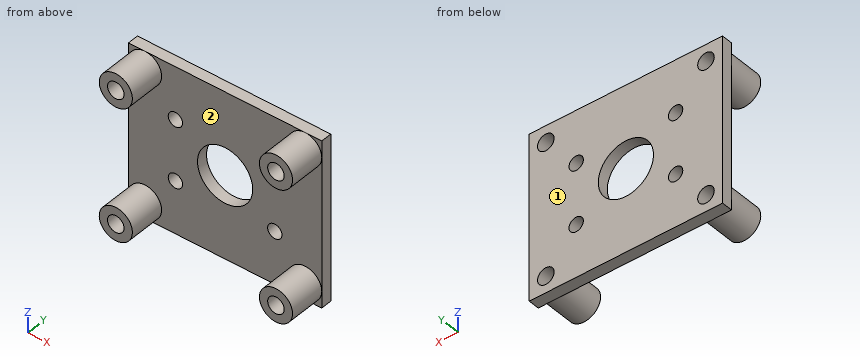
```python
from build123d import *

# Parameters (mm, degrees)
SKETCH1_W           = 35
SKETCH1_H           = 30
BOSS_EXTRUDE1_DEPTH = 2
CUT_EXTRUDE1_REACH  = 25.135
SKETCH2_R           = 1.3
CUT_EXTRUDE2_REACH  = 25.135
SKETCH3_R           = 1.5
SKETCH4_R           = 3
BOSS_EXTRUDE2_DEPTH = 6.5
CUT_EXTRUDE3_REACH  = 25.948
SKETCH5_R           = 1.5
SKETCH7_R           = 5
CUT_EXTRUDE4_DEPTH  = 3


with BuildPart() as part:
    # Sketch1 → Boss-Extrude1 (new body)
    with BuildSketch(Plane(origin=(0, 0, 0), x_dir=(1, 0, 0), z_dir=(0, 1, 0))):
        Rectangle(SKETCH1_W, SKETCH1_H)
    extrude(amount=BOSS_EXTRUDE1_DEPTH)

    # Sketch2 → Cut-Extrude1 (cut, up to next)
    with BuildSketch(Plane(origin=(0, 2, 0), x_dir=(1, 0, 0), z_dir=(0, 1, 0)), mode=Mode.PRIVATE) as cut_extrude1_sk1:
        with Locations(Location((9, 5.5, 0), (0, 0, 270))):
            Circle(SKETCH2_R)
    cut_extrude1_tool1 = extrude(cut_extrude1_sk1.sketch, amount=-CUT_EXTRUDE1_REACH, mode=Mode.PRIVATE) & part.part
    # Sketch2 → Cut-Extrude1 (cut, up to next)
    with BuildSketch(Plane(origin=(0, 2, 0), x_dir=(1, 0, 0), z_dir=(0, 1, 0)), mode=Mode.PRIVATE) as cut_extrude1_sk2:
        with Locations(Location((-9, 5.5, 0), (0, 0, 270))):
            Circle(SKETCH2_R)
    cut_extrude1_tool2 = extrude(cut_extrude1_sk2.sketch, amount=-CUT_EXTRUDE1_REACH, mode=Mode.PRIVATE) & part.part
    # Sketch2 → Cut-Extrude1 (cut, up to next)
    with BuildSketch(Plane(origin=(0, 2, 0), x_dir=(1, 0, 0), z_dir=(0, 1, 0)), mode=Mode.PRIVATE) as cut_extrude1_sk3:
        with Locations(Location((9, -5.5, 0), (0, 0, 270))):
            Circle(SKETCH2_R)
    cut_extrude1_tool3 = extrude(cut_extrude1_sk3.sketch, amount=-CUT_EXTRUDE1_REACH, mode=Mode.PRIVATE) & part.part
    # Sketch2 → Cut-Extrude1 (cut, up to next)
    with BuildSketch(Plane(origin=(0, 2, 0), x_dir=(1, 0, 0), z_dir=(0, 1, 0)), mode=Mode.PRIVATE) as cut_extrude1_sk4:
        with Locations(Location((-9, -5.5, 0), (0, 0, 270))):
            Circle(SKETCH2_R)
    cut_extrude1_tool4 = extrude(cut_extrude1_sk4.sketch, amount=-CUT_EXTRUDE1_REACH, mode=Mode.PRIVATE) & part.part
    add(cut_extrude1_tool1.solids().sort_by_distance((9, 2, -5.5))[0], mode=Mode.SUBTRACT)
    add(cut_extrude1_tool2.solids().sort_by_distance((-9, 2, -5.5))[0], mode=Mode.SUBTRACT)
    add(cut_extrude1_tool3.solids().sort_by_distance((9, 2, 5.5))[0], mode=Mode.SUBTRACT)
    add(cut_extrude1_tool4.solids().sort_by_distance((-9, 2, 5.5))[0], mode=Mode.SUBTRACT)

    # Sketch3 → Cut-Extrude2 (cut, up to next)
    with BuildSketch(Plane.XZ, mode=Mode.PRIVATE) as cut_extrude2_sk1:
        with Locations(Location((-14.5, 12, 0), (0, 0, 270))):
            Circle(SKETCH3_R)
    cut_extrude2_tool1 = extrude(cut_extrude2_sk1.sketch, amount=-CUT_EXTRUDE2_REACH, mode=Mode.PRIVATE) & part.part
    # Sketch3 → Cut-Extrude2 (cut, up to next)
    with BuildSketch(Plane.XZ, mode=Mode.PRIVATE) as cut_extrude2_sk2:
        with Locations(Location((14.5, 12, 0), (0, 0, 270))):
            Circle(SKETCH3_R)
    cut_extrude2_tool2 = extrude(cut_extrude2_sk2.sketch, amount=-CUT_EXTRUDE2_REACH, mode=Mode.PRIVATE) & part.part
    # Sketch3 → Cut-Extrude2 (cut, up to next)
    with BuildSketch(Plane.XZ, mode=Mode.PRIVATE) as cut_extrude2_sk3:
        with Locations(Location((14.5, -12, 0), (0, 0, 90))):
            Circle(SKETCH3_R)
    cut_extrude2_tool3 = extrude(cut_extrude2_sk3.sketch, amount=-CUT_EXTRUDE2_REACH, mode=Mode.PRIVATE) & part.part
    # Sketch3 → Cut-Extrude2 (cut, up to next)
    with BuildSketch(Plane.XZ, mode=Mode.PRIVATE) as cut_extrude2_sk4:
        with Locations(Location((-14.5, -12, 0), (0, 0, 90))):
            Circle(SKETCH3_R)
    cut_extrude2_tool4 = extrude(cut_extrude2_sk4.sketch, amount=-CUT_EXTRUDE2_REACH, mode=Mode.PRIVATE) & part.part
    add(cut_extrude2_tool1.solids().sort_by_distance((-14.5, 0, 12))[0], mode=Mode.SUBTRACT)
    add(cut_extrude2_tool2.solids().sort_by_distance((14.5, 0, 12))[0], mode=Mode.SUBTRACT)
    add(cut_extrude2_tool3.solids().sort_by_distance((14.5, 0, -12))[0], mode=Mode.SUBTRACT)
    add(cut_extrude2_tool4.solids().sort_by_distance((-14.5, 0, -12))[0], mode=Mode.SUBTRACT)

    # Sketch4 → Boss-Extrude2 (add)
    with BuildSketch(Plane.XZ):
        with Locations(Location((-14.5, 12, 0), (0, 0, 90))):
            Circle(SKETCH4_R)
        with Locations(Location((14.5, 12, 0), (0, 0, 90))):
            Circle(SKETCH4_R)
        with Locations(Location((-14.5, -12, 0), (0, 0, 270))):
            Circle(SKETCH4_R)
        with Locations(Location((14.5, -12, 0), (0, 0, 270))):
            Circle(SKETCH4_R)
    extrude(amount=BOSS_EXTRUDE2_DEPTH)

    # Sketch5 → Cut-Extrude3 (cut, up to next)
    with BuildSketch(Plane(origin=(0, 0, 0), x_dir=(1, 0, 0), z_dir=(0, 1, 0)), mode=Mode.PRIVATE) as cut_extrude3_sk1:
        with Locations(Location((-14.5, 12, 0), (0, 0, 90))):
            Circle(SKETCH5_R)
    cut_extrude3_tool1 = extrude(cut_extrude3_sk1.sketch, amount=-CUT_EXTRUDE3_REACH, mode=Mode.PRIVATE) & part.part
    # Sketch5 → Cut-Extrude3 (cut, up to next)
    with BuildSketch(Plane(origin=(0, 0, 0), x_dir=(1, 0, 0), z_dir=(0, 1, 0)), mode=Mode.PRIVATE) as cut_extrude3_sk2:
        with Locations(Location((14.5, 12, 0), (0, 0, 90))):
            Circle(SKETCH5_R)
    cut_extrude3_tool2 = extrude(cut_extrude3_sk2.sketch, amount=-CUT_EXTRUDE3_REACH, mode=Mode.PRIVATE) & part.part
    # Sketch5 → Cut-Extrude3 (cut, up to next)
    with BuildSketch(Plane(origin=(0, 0, 0), x_dir=(1, 0, 0), z_dir=(0, 1, 0)), mode=Mode.PRIVATE) as cut_extrude3_sk3:
        with Locations(Location((14.5, -12, 0), (0, 0, 90))):
            Circle(SKETCH5_R)
    cut_extrude3_tool3 = extrude(cut_extrude3_sk3.sketch, amount=-CUT_EXTRUDE3_REACH, mode=Mode.PRIVATE) & part.part
    # Sketch5 → Cut-Extrude3 (cut, up to next)
    with BuildSketch(Plane(origin=(0, 0, 0), x_dir=(1, 0, 0), z_dir=(0, 1, 0)), mode=Mode.PRIVATE) as cut_extrude3_sk4:
        with Locations(Location((-14.5, -12, 0), (0, 0, 90))):
            Circle(SKETCH5_R)
    cut_extrude3_tool4 = extrude(cut_extrude3_sk4.sketch, amount=-CUT_EXTRUDE3_REACH, mode=Mode.PRIVATE) & part.part
    add(cut_extrude3_tool1.solids().sort_by_distance((-14.5, 0, -12))[0], mode=Mode.SUBTRACT)
    add(cut_extrude3_tool2.solids().sort_by_distance((14.5, 0, -12))[0], mode=Mode.SUBTRACT)
    add(cut_extrude3_tool3.solids().sort_by_distance((14.5, 0, 12))[0], mode=Mode.SUBTRACT)
    add(cut_extrude3_tool4.solids().sort_by_distance((-14.5, 0, 12))[0], mode=Mode.SUBTRACT)

    # Sketch7 → Cut-Extrude4 (cut)
    with BuildSketch(Plane(origin=(0, 2, 0), x_dir=(1, 0, 0), z_dir=(0, 1, 0))):
        with Locations(Location((0, 0, 0), (0, 0, 270))):
            Circle(SKETCH7_R)
    extrude(amount=-CUT_EXTRUDE4_DEPTH, mode=Mode.SUBTRACT)


solid = part.part
```
Model file for the job. Use its own axes, mm. Face numbers are marked on the shaded views. Coordinates: 2 decimals unless noted, no trailing zeros. Loops run counter-clockwise (first coordinate to the right, second up) from the corner with the lowest first, then second, coordinate; pieces in that order, holes last. Notation, with made-up numbers: (-11.75, -18) - (43.25, -18) arc R30 ccw to (43.25, 10) - close; hole circle Ø11 at (72.5, -24.75). An arc over 180 degrees is marked (long way). Answer as a JSON object with one key per item and string values. Group by question number.
(1) Cut at B-B (x = -9). Give the cut face in (y, z), then the cut area to 3 significant figures.
(2) Two-plate mould, pull along Z, no slides. Class the marked faces 1 and 2: released by +Z, released by -Z, zero draft, split by the parting line, or undercut.
(3) Cut at A-A (y = -2.5). Give the cut face in (x, z), then the cut area to 3 significant figures.
(4) Flat gauge pin, fed straight in: pin 1 (4 mm diameter, centred on x = -13.5, z = -3, fed in from -Y). Where does the tip first touch, or does it go through?
(5) Cut at D-D (x = 0). Give the cut face in (y, z).
(6) Cut at C-C (z = 0). Give the cut face in (x, y).
(7) Probe line 1 along X through (y, z) = (0.7, 5.5); line 2 along X through (y, z) = (-4, 12); line 3 along Z through (x, y) = (-14.5, 0.25). List the from-to ranges inside material, lowest first.
Geometry says:
{
 "1": {"outline": "(0, -15) - (2, -15) - (2, -6.8) - (0, -6.8) - close; (0, -4.2) - (2, -4.2) - (2, 4.2) - (0, 4.2) - close; (0, 6.8) - (2, 6.8) - (2, 15) - (0, 15) - close", "area": "49.6 mm^2"},
 "2": {"face 1": "zero draft", "face 2": "undercut"},
 "3": {"outline": "circle Ø6 at (-14.5, -12); circle Ø6 at (-14.5, 12); circle Ø6 at (14.5, -12); circle Ø6 at (14.5, 12); hole circle Ø3 at (-14.5, -12); hole circle Ø3 at (-14.5, 12); hole circle Ø3 at (14.5, -12); hole circle Ø3 at (14.5, 12)", "area": "84.8 mm^2"},
 "4": {"pin 1": "stops at y = 0"},
 "5": {"outline": "(0, -15) - (2, -15) - (2, -5) - (0, -5) - close; (0, 5) - (2, 5) - (2, 15) - (0, 15) - close"},
 "6": {"outline": "(-17.5, 0) - (-5, 0) - (-5, 2) - (-17.5, 2) - close; (5, 0) - (17.5, 0) - (17.5, 2) - (5, 2) - close"},
 "7": {"line 1": "x = -17.5 to -10.3, -7.7 to 7.7, 10.3 to 17.5", "line 2": "x = -17.5 to -16, -13 to -11.5, 11.5 to 13, 16 to 17.5", "line 3": "z = -15 to -13.5, -10.5 to 10.5, 13.5 to 15"}
}
